Design review of the part built by this model. Coordinates are the model's own, in mm. A direction names the side the tool comes from. Coordinates: 2 decimals unless noted, no trailing zeros. Write each loop counter-clockwise with the first axis right and the second up, starting at its lowest first coordinate (ties: lowest second). Pieces come first, ordered by that corner, then holes. Notation, with made-up numbers: (42, 86) - (80, 86) arc R24 cw to (80, 96) - close; hole circle Ø2 at (13.5, -38.5). An arc over 180 degrees is marked (long way). Answer as a JSON object with one key per item and string values.
Autodesk Inventor part; units mm, degrees
ref_plane "MSC_PF1" through (0, 0, 0) normal (0, 1, 0) x (-1, 0, 0)
ref_plane "MSC_PT1" through (0, 0, -11.7108) normal (0, 0, -1) x (-1, 0, 0)
ref_plane "YZ Plane" through (0, 0, 0) normal (1, 0, 0) x (0, 1, 0)
sketch "Sketch2" plane through (0, 0, 0) normal (0, 1, 0) x (-1, 0, 0)
  line L0 (0, -11.7108) -> (0, -36.7108)
  line L1 (0, -36.7108) -> (2.1, -36.7108)
  line L2 (2.5, -36.3108) -> (2.5, -20.7108)
  line L3 (2.5, -20.7108) -> (2.2, -20.1912)
  line L4 (2.2, -20.1912) -> (2.2, -11.7108)
  line L5 (2.2, -11.7108) -> (0, -11.7108)
  line L6 (2.1, -36.7108) -> (2.5, -36.3108)
  line L7 (2.5, -36.7108) -> (2.5, -37.2765)
  line L8 (0, -42.3897) -> (0, -6.5977)
  dimension "Ds" = 4.4
  dimension "NND" = 5
  dimension "b" = 16
  dimension "d3" = 30
  dimension "d5" = 45
  dimension "PTC" = 0.8
  dimension "NLG" = 25
revolve "Revolution1" add sketch "Sketch2" angle 360 about axis through (0, 0, -11.7108) along (0, 0, -1)
sketch "Sketch3" plane through (0, 0, -11.7108) normal (0, 0, 1) x (1, 0, 0)
  circle A0 centre (0, 0) radius 2.2
  line L0 (0, 4) -> (2.3094, 4)
  line L1 (2.3094, 4) -> (4.6188, 0)
  line L2 (4.6188, 0) -> (0, 0)
  line L3 (0, 0) -> (0, 4)
  line L4 (0, 4) -> (-2.3094, 4)
  line L5 (-2.3094, 4) -> (-4.6188, 0)
  line L6 (0, -4) -> (2.3094, -4)
  line L7 (2.3094, -4) -> (4.6188, 0)
  line L8 (-2.3094, -4) -> (-4.6188, 0)
  line L9 (0, -4) -> (-2.3094, -4)
  dimension "d9" = 60
  dimension "ParS" = 8
  dimension "msp_d11" = 8
extrude "Extrusion1" add sketch "Sketch3" along normal blind 3.5
sketch "Sketch4" plane through (0, 0, 0) normal (0, 1, 0) x (-1, 0, 0)
  line L0 (-4, -8.2108) -> (-4.6188, -8.2108)
  line L1 (-4.6188, -8.2108) -> (-4.6188, -8.5681)
  line L2 (-4.6188, -8.5681) -> (-4, -8.2108)
  line L3 (0, -19.5602) -> (0, 35.3854)
  line L4 (0, 27.536) -> (0, 27.1787)
  line L5 (-4.6188, -11.7108) -> (-4.6188, -8.2108)
  line L6 (-2.3094, -8.2108) -> (-4.6188, -8.2108)
  dimension "d14" = 30
  dimension "msp_d15" = 8
revolve "Revolution2" cut sketch "Sketch4" angle 360 about axis through (0, 0, 27.536) along (0, 0, -1)
sketch "Sketch5" plane through (0, 0, -8.2108) normal (0, 0, 1) x (1, 0, 0)
  arc A0 (3.4641, 2) -> (0, 4) centre (0, 0) ccw
  circle A1 centre (0, 0) radius 3
  dimension "d27" = 6
extrude "Extrusion2" cut sketch "Sketch5" against normal blind 0.7
thread "Thread1"
ref_plane "MSC_PF1" through (0, 0, 0) normal (0, 1, 0) x (-1, 0, 0)
ref_plane "MSC_PT1" through (0, 0, -11.7108) normal (0, 0, -1) x (-1, 0, 0)
fillet "Fillet1" radius 0.2 1 edges at (2.2, 0, -11.7108)
equation "\"msp_d11\" = ParS"
equation "\"msp_d15\" = ParS"
equation "\"d27\" = 0.75 * ParS"
equation "\"d28\" = 0.2 * ParK"
equation "\"d30\" = r"
equation "\"msp_d17\" = b"
equation "\"r\" = 0.2"
equation "\"THREADDIA\" = NND"
properties part number "ISO 4015 - M5 x 25" material "Stainless Steel, 440C"
(1) Take a section at A-A, the plane z = -32.75. Write out the cut boundary in (x, y), and give its area (3 significant figures).
Solved:
{"outline": "circle Ø5 at (0, 0)", "area": "19.6 mm^2"}
(2) For pin 1 (1 mm diameter, centred on x = 0, z = -29.5, fed in from -Y); pin 2 (1.5 mm diameter, centred on y = 3, z = -31.5, fed in from -X); pin 3 (5 mm diameter, centred on x = 1.5, z = -19, fed in from +Y), all flat-tipped, find the tip position at first contact; note any pin that passes through.
Solved:
{"pin 1": "stops at y = -2.5", "pin 2": "stops at x = -1.09", "pin 3": "stops at y = 2.5"}
(3) To check wall thickness, follow line 1 (Y direction, x = 0, z = -8.65); line 2 (Z direction, x = -2, y = 3); line 3 (Z direction, x = -0.25, y = -1.75). State the ranges of each line that lie inside material, in increasing order. Write a range as from..to.
Solved:
{"line 1": "y = -4..-3, 3..4", "line 2": "z = -11.71..-8.21", "line 3": "z = -36.71..-8.91"}
(4) The part is to be moulded in two halves that separate along Z. For faces 4 (the face through (2.084, -3.589, -8.298)), 5 (the face through (-2.1, -0.66, -15.99)), 6 (the face through (3.448, 2.028, -9.985)), say which applies: pulls with the +Z half, pulls with the -Z half, needs draft (parallel to the pull), parting line crosses it, or undercut.
Solved:
{"face 4": "pulls with the +Z half", "face 5": "undercut", "face 6": "needs draft"}
(5) Tool access review of faces 1 (the face through (1, 3, -8.211)), 2 (the face through (-3, 0.1, -8.6)), 3 (the face through (0.54, 2.44, -28.4)): name each direction out of +Z, -Z, +X, -X, +Y, -Y from which nothing blocks a thin tool from reaching the whole face with its end or side.
Solved:
{"face 1": "+Z, +X, -X, +Y, -Y", "face 2": "+Z", "face 3": "-Z"}
(6) Take a section at B-B, the plane z = -18.25. Write out the cut boundary in (x, y).
Solved:
{"outline": "circle Ø4.4 at (0, 0)"}
